Build history of the part. All positions in model axes, mm. A direction names the side the tool comes from. Round coordinates to 2 decimals unless told otherwise and drop trailing zeros. Loops run counter-clockwise (first coordinate to the right, second up) from the corner with the lowest first, then second, coordinate; pieces in that order, holes last. Notation, with made-up numbers: (-15.5, -12.75) - (-3.5, -12.75) arc R20 ccw to (-3.5, 20.25) - close; hole circle Ø10 at (65, 59.25). An arc over 180 degrees is marked (long way). Use one line per item in the form item = value. Start each with the question number.
Q1. Saw through at B-B (z = 0). Give the cut face in (x, y).
Q2. Pin check, flat tips, straight feed: pin 1 (3 mm diameter, centred on y = 13.5, z = 73.5, fed in from +X); pin 2 (12 mm diameter, centred on y = 16, z = 455.5, fed in from +X); pin 3 (2 mm diameter, centred on x = -513, y = 7.5, fed in from +Z). Stop position of each tip, or through.
Q3. 3-axis set-ups, long thin cutter, end or side, ignore diameter. For faces 1 (the face through (-7.153, 5.963, -153.854)), 2 (the face through (-1290, 0, -377)): which of +Z, -Z, +X, -X, +Y, -Y reach the whole face in a straight line?
Q4. Drill centre lines: line 1 (X direction, y = 27, z = 0); line 2 (X direction, y = 10, z = 0); line 3 (Z direction, x = -823.5, y = 28.5). Where is each one in solid material? Low to high.
Q5. Saw through at A-A (x = -700). Give the cut face in (y, z).
Q6. Mould opens along Y. For faces 3 (the face through (-61.24, 38.92, 332.24)), 4 (the face through (-1077, 40, 590)), 5 (the face through (-7.272, 34.017, -153.828)), 6 (the face through (-1399, 19.87, -91.78)) say: released by +Y, released by -Y, zero draft, split by the parting line, or undercut.
```python
from build123d import *


with BuildPart() as part:
    # Sketch1 → Revolve1 (revolve)
    with BuildSketch(Plane.XY, mode=Mode.PRIVATE) as revolve1_sk:
        with BuildLine():
            Line((0, 0), (0, 40))
            Line((0, 40), (20, 40))
            Line((20, 40), (20, 37.86788351))
            ThreePointArc((20, 37.86788351), (19.407559514, 36.251957552), (17.91102664, 35.401903562))
            Line((17.91102664, 35.401903562), (9.17794672, 33.946284063))
            ThreePointArc((9.17794672, 33.946284063), (6.184880972, 32.246176083), (5, 29.014324168))
            Line((5, 29.014324168), (5, 10.985675832))
            ThreePointArc((5, 10.985675832), (6.184880972, 7.753823917), (9.17794672, 6.053715937))
            Line((9.17794672, 6.053715937), (17.91102664, 4.598096438))
            ThreePointArc((17.91102664, 4.598096438), (19.407559514, 3.748042448), (20, 2.13211649))
            Line((20, 2.13211649), (20, 0))
            Line((20, 0), (0, 0))
        make_face()
    revolve(revolve1_sk.sketch.rotate(Axis((-700, 40, 0), (0, -1, 0)), 90), axis=Axis((-700, 40, 0), (0, -1, 0)))


solid = part.part
```
Report:
q1.outline = (-1420, 0) - (-1400, 0) - (-1400, 40) - (-1420, 40) - (-1420, 37.87) arc R2.5 ccw to (-1417.91, 35.4) - (-1409.18, 33.95) arc R5 cw to (-1405, 29.01) - (-1405, 10.99) arc R5 cw to (-1409.18, 6.05) - (-1417.91, 4.6) arc R2.5 ccw to (-1420, 2.13) - close; (0, 0) - (20, 0) - (20, 2.13) arc R2.5 ccw to (17.91, 4.6) - (9.18, 6.05) arc R5 cw to (5, 10.99) - (5, 29.01) arc R5 cw to (9.18, 33.95) - (17.91, 35.4) arc R2.5 ccw to (20, 37.87) - (20, 40) - (0, 40) - close
q2.pin_1 = 1.31
q2.pin_2 = -156.88
q2.pin_3 = 682.66
q3.face_1 = none
q3.face_2 = +Z, -Z, +X, -X, -Y
q4.line_1 = -1405 to -1400, 0 to 5
q4.line_2 = -1405.1 to -1400, 0 to 5.1
q4.line_3 = -694.1 to -689.02, 689.02 to 694.1
q5.outline = (0, -720) - (2.13, -720) arc R2.5 ccw to (4.6, -717.91) - (6.05, -709.18) arc R5 cw to (10.99, -705) - (29.01, -705) arc R5 cw to (33.95, -709.18) - (35.4, -717.91) arc R2.5 ccw to (37.87, -720) - (40, -720) - (40, -700) - (0, -700) - close; (0, 700) - (40, 700) - (40, 720) - (37.87, 720) arc R2.5 ccw to (35.4, 717.91) - (33.95, 709.18) arc R5 cw to (29.01, 705) - (10.99, 705) arc R5 cw to (6.05, 709.18) - (4.6, 717.91) arc R2.5 ccw to (2.13, 720) - (0, 720) - close
q6.face_3 = zero draft
q6.face_4 = released by +Y
q6.face_5 = undercut
q6.face_6 = undercut
